```python
from build123d import *

# Parameters (mm, degrees)
SKETCH1_R                = 2.5
BOSS_EXTRUDE1_DEPTH      = 4
BOSS_EXTRUDE3_DEPTH      = 8
BOSS_EXTRUDE3_DEPTH_BACK = 8
SKETCH3_R                = 5
SKETCH3_R_2              = 2.5
CUT_EXTRUDE1_START       = -10
CUT_EXTRUDE1_DEPTH       = 10


with BuildPart() as part:
    # Sketch1 → Boss-Extrude1 (new body)
    with BuildSketch(Plane(origin=(0, 0, 0), x_dir=(1, 0, 0), z_dir=(0, 1, 0))):
        with BuildLine():
            Line((0, 5), (30, 5))
            ThreePointArc((30, 5), (35, 0), (30, -5))
            Line((30, -5), (0, -5))
            ThreePointArc((0, -5), (-5, 0), (0, 5))
        make_face()
        with Locations(Location((0, 0, 0), (0, 0, 270))):
            Circle(SKETCH1_R, mode=Mode.SUBTRACT)
        with Locations(Location((30, 0, 0), (0, 0, 270))):
            Circle(SKETCH1_R, mode=Mode.SUBTRACT)
    extrude(amount=BOSS_EXTRUDE1_DEPTH)

    # Sketch3 → Boss-Extrude3 (add, two sides: drawn at the far end of the back side and taken through both)
    with BuildSketch(Plane(origin=(0, 2, 0), x_dir=(1, 0, 0), z_dir=(0, 1, 0)).offset(-BOSS_EXTRUDE3_DEPTH_BACK)):
        with Locations(Location((30, 0, 0), (0, 0, 270))):
            Circle(SKETCH3_R)
        with Locations(Location((30, 0, 0), (0, 0, 270))):
            Circle(SKETCH3_R_2, mode=Mode.SUBTRACT)
    extrude(amount=BOSS_EXTRUDE3_DEPTH + BOSS_EXTRUDE3_DEPTH_BACK)

    # Sketch4 → Cut-Extrude1 (cut)
    with BuildSketch(Plane(origin=(0, 4, 0), x_dir=(1, 0, 0), z_dir=(0, 1, 0)).offset(CUT_EXTRUDE1_START)):
        with BuildLine():
            Line((0, -5), (30, -5))
            ThreePointArc((30, -5), (28.552126, -4.785777), (27.228319, -4.161464))
            add(Edge.make_bspline(
                [(2.771681, -4.161464), (6.847787, -3.053821), (15, -1.946179), (23.152213, -3.053821), (27.228319, -4.161464)],
                knots=[0.092389, 0.092389, 0.092389, 0.092389, 0.5, 0.907611, 0.907611, 0.907611, 0.907611], degree=3))
            ThreePointArc((2.771681, -4.161464), (1.447874, -4.785777), (0, -5))
        make_face()
        with BuildLine():
            Line((0, 5), (30, 5))
            ThreePointArc((30, 5), (28.552126, 4.785777), (27.228319, 4.161464))
            add(Edge.make_bspline(
                [(2.771681, 4.161464), (6.847787, 3.053821), (15, 1.946179), (23.152213, 3.053821), (27.228319, 4.161464)],
                knots=[0.092389, 0.092389, 0.092389, 0.092389, 0.5, 0.907611, 0.907611, 0.907611, 0.907611], degree=3))
            ThreePointArc((2.771681, 4.161464), (1.447874, 4.785777), (0, 5))
        make_face()
    extrude(amount=CUT_EXTRUDE1_DEPTH, mode=Mode.SUBTRACT)


solid = part.part
```
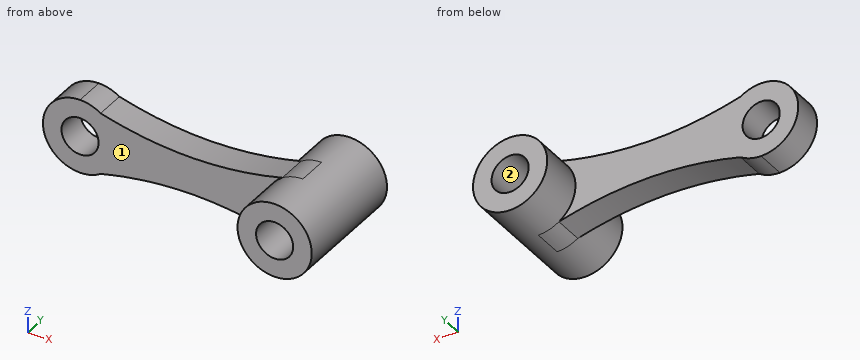
The model under review builds one solid part; all positions refer to its coordinate system, in mm. Face numbers are marked on the shaded views. Round coordinates to 2 decimals unless told otherwise and drop trailing zeros. Write each loop counter-clockwise with the first axis right and the second up, starting at its lowest first coordinate (ties: lowest second). Pieces come first, ordered by that corner, then holes.
(1) Wall thickness on L1, parallel to X at y = 2.55, z = 0; L2, parallel to X at y = 5.25, z = 0; L3, parallel to X at y = -1.5, z = 1: over which ranges is each line inside the solid? List them lowest first.
(2) We need section C-C on y = 0.5. Give the number of separate pieces and of enclosed holes in the cut face, and give its area (3 significant figures).
(3) Insertion check: pin 1 (3 mm diameter, centred on x = 17.5, z = -3, fed in from -Y); pin 2 (1.5 mm diameter, centred on y = 8, z = -3.5, fed in from -X); pin 3 (3 mm diameter, centred on x = 4.5, z = -1, fed in from +Y); pin 4 (5 mm diameter, centred on x = 8, y = -3.5, fed in from +Z). Each pin has a flat end and moves straight along its axis. Give the tip position at first contact, or say it passes through.
(4) We need section B-B on y = 8.25. Give the boundary of the cut face in (x, z).
(5) Mouldability with a two-part tool opening along X and no side actions: class the marked faces 1 and 2 as +X half, -X half, draft (parallel to the pull), parting line (faces both ways), or undercut.
(6) We need section D-D on z = -1.75. Give the boundary of the cut face in (x, y).
(7) We need section A-A on z = 0. Give the boundary of the cut face in (x, y).
Findings below:
1. L1: x = -5 to -2.5, 2.5 to 27.5, 32.5 to 35
1. L2: x = 25 to 27.5, 32.5 to 35
1. L3: x = 25.1 to 27.71, 32.29 to 34.9
2. separate pieces: 1
2. enclosed holes: 2
2. area: 241 mm2
3. pin 1: stops at y = 0
3. pin 2: stops at x = 25.82
3. pin 3: stops at y = 4
3. pin 4: passes through
4. outline: circle Ø10 at (30, 0); hole circle Ø5 at (30, 0)
5. face 1: draft
5. face 2: undercut
6. outline: (-4.68, 0) - (-1.79, 0) - (-1.79, 4) - (-4.68, 4) - close; (1.79, 0) - (25.32, 0) - (25.32, -6) - (28.21, -6) - (28.21, 10) - (25.32, 10) - (25.32, 4) - (1.79, 4) - close; (31.79, -6) - (34.68, -6) - (34.68, 10) - (31.79, 10) - close
7. outline: (-5, 0) - (-2.5, 0) - (-2.5, 4) - (-5, 4) - close; (2.5, 0) - (25, 0) - (25, -6) - (27.5, -6) - (27.5, 10) - (25, 10) - (25, 4) - (2.5, 4) - close; (32.5, -6) - (35, -6) - (35, 10) - (32.5, 10) - close
